Check sheet for the modelled part. Datum: model origin and axes. Units: mm. Round coordinates to 2 decimals unless told otherwise and drop trailing zeros. Write each loop counter-clockwise with the first axis right and the second up, starting at its lowest first coordinate (ties: lowest second). Pieces come first, ordered by that corner, then holes. Notation, with made-up numbers: (56.25, -26) -> (67.25, -26) arc R29 cw to (67.25, 3) -> close; hole circle Ø5 at (19.5, -17). An arc over 180 degrees is marked (long way). One line per item, written item: value.
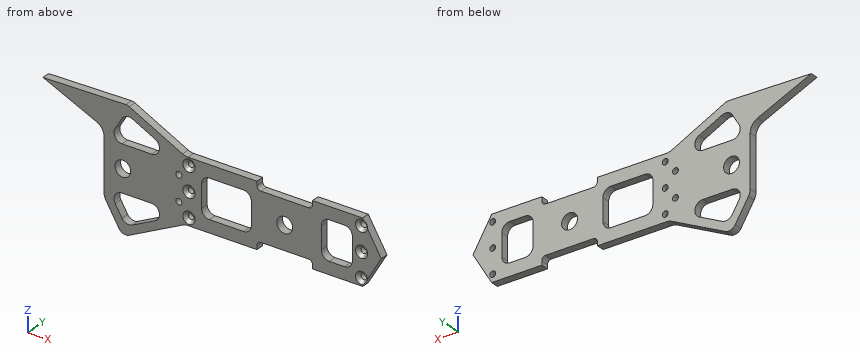
from build123d import *

# Parameters (mm, degrees)
CROQUIS1_R              = 6.35
SALIENTE_EXTRUIR1_DEPTH = 6.35
REDONDEO1_R             = 10
CORTAR_EXTRUIR2_DEPTH   = 225.405229946
CORTAR_EXTRUIR3_DEPTH   = 225.405229946
CROQUIS7_R              = 2.38125
CORTAR_EXTRUIR4_DEPTH   = 225.405229946
CROQUIS8_R              = 2.38125
CORTAR_EXTRUIR5_DEPTH   = 225.405229946
CHAFL_N1_SIZE           = 2.5


with BuildPart() as part:
    # Croquis1 → Saliente-Extruir1 (new body)
    with BuildSketch(Plane(origin=(0, 0, 0), x_dir=(1, 0, 0), z_dir=(0, 1, 0))):
        with BuildLine():
            Line((37.5, -25.4), (52.5, 0))
            Line((52.5, 0), (37.5, 25.4))
            Line((37.5, 25.4), (-105, 25.4))
            Line((-105, 25.4), (-149.746813481, 47.731727951))
            ThreePointArc((-149.746813481, 47.731727951), (-154.357530471, 48.146831931), (-158.024774803, 45.321528145))
            Line((-158.024774803, 45.321528145), (-170, 25.4))
            Line((-170, 25.4), (-170, -25.4))
            Line((-170, -25.4), (-219.03156103, -47.147007635))
            Line((-219.03156103, -47.147007635), (-152.702210171, -48.398869348))
            ThreePointArc((-152.702210171, -48.398869348), (-151.184140049, -48.244143221), (-149.746813481, -47.731727951))
            Line((-149.746813481, -47.731727951), (-105, -25.4))
            Line((-105, -25.4), (37.5, -25.4))
        make_face()
        with Locations(Location((-155, 0, 0), (0, 0, 270))):
            Circle(CROQUIS1_R, mode=Mode.SUBTRACT)
        with Locations(Location((-25, 0, 0), (0, 0, 270))):
            Circle(CROQUIS1_R, mode=Mode.SUBTRACT)
        with BuildLine():
            Line((-129.045100716, 30.303281185), (-147.329198773, 39.428299747))
            ThreePointArc((-147.329198773, 39.428299747), (-151.939915763, 39.843403727), (-155.607160095, 37.018099941))
            Line((-155.607160095, 37.018099941), (-161.092389512, 27.893081378))
            ThreePointArc((-161.092389512, 27.893081378), (-161.177056347, 21.495189828), (-155.65, 18.271553233))
            Line((-155.65, 18.271553233), (-131.880672526, 18.271553233))
            ThreePointArc((-131.880672526, 18.271553233), (-125.699998109, 23.164925706), (-129.045100716, 30.303281185))
        make_face(mode=Mode.SUBTRACT)
        with BuildLine():
            Line((-129.045100716, -30.303281185), (-147.329198773, -39.428299747))
            ThreePointArc((-147.329198773, -39.428299747), (-151.939915763, -39.843403727), (-155.607160095, -37.018099941))
            Line((-155.607160095, -37.018099941), (-161.092389512, -27.893081378))
            ThreePointArc((-161.092389512, -27.893081378), (-161.177056347, -21.495189828), (-155.65, -18.271553233))
            Line((-155.65, -18.271553233), (-131.880672526, -18.271553233))
            ThreePointArc((-131.880672526, -18.271553233), (-125.699998109, -23.164925706), (-129.045100716, -30.303281185))
        make_face(mode=Mode.SUBTRACT)
    extrude(amount=SALIENTE_EXTRUIR1_DEPTH)

    # Redondeo1
    redondeo1_edges = [part.edges().sort_by_distance(p)[0] for p in [
        (-105, 3.175, -25.4),
        (-170, 3.175, -25.4),
        (-170, 3.175, 25.4),
        (-105, 3.175, 25.4),
    ]]
    fillet(redondeo1_edges, radius=REDONDEO1_R)

    # Croquis5 → Cortar-Extruir2 (cut, through all)
    with BuildSketch(Plane.XZ):
        with BuildLine():
            Line((-5.875, 19.05), (-44.125, 19.05))
            ThreePointArc((-44.125, 19.05), (-46.37006403, 19.97993597), (-47.3, 22.225))
            Line((-47.3, 22.225), (-47.3, 25.4))
            Line((-47.3, 25.4), (-44.125, 25.4))
            Line((-44.125, 25.4), (-5.875, 25.4))
            Line((-5.875, 25.4), (-2.7, 25.4))
            Line((-2.7, 25.4), (-2.7, 22.225))
            ThreePointArc((-2.7, 22.225), (-3.62993597, 19.97993597), (-5.875, 19.05))
        make_face()
        with BuildLine():
            Line((-5.875, -19.05), (-44.125, -19.05))
            ThreePointArc((-44.125, -19.05), (-46.37006403, -19.97993597), (-47.3, -22.225))
            Line((-47.3, -22.225), (-47.3, -25.4))
            Line((-47.3, -25.4), (-44.125, -25.4))
            Line((-44.125, -25.4), (-5.875, -25.4))
            Line((-5.875, -25.4), (-2.7, -25.4))
            Line((-2.7, -25.4), (-2.7, -22.225))
            ThreePointArc((-2.7, -22.225), (-3.62993597, -19.97993597), (-5.875, -19.05))
        make_face()
    extrude(amount=-CORTAR_EXTRUIR2_DEPTH, mode=Mode.SUBTRACT)

    # Croquis6 → Cortar-Extruir3 (cut, through all)
    with BuildSketch(Plane.XZ):
        with BuildLine():
            Line((-85.475, 15.4), (-58.175, 15.4))
            ThreePointArc((-58.175, 15.4), (-53.684871939, 13.540128061), (-51.825, 9.05))
            Line((-51.825, 9.05), (-51.825, -9.05))
            ThreePointArc((-51.825, -9.05), (-53.684871939, -13.540128061), (-58.175, -15.4))
            Line((-58.175, -15.4), (-85.475, -15.4))
            ThreePointArc((-85.475, -15.4), (-89.965128061, -13.540128061), (-91.825, -9.05))
            Line((-91.825, -9.05), (-91.825, 9.05))
            ThreePointArc((-91.825, 9.05), (-89.965128061, 13.540128061), (-85.475, 15.4))
        make_face()
        with BuildLine():
            Line((10.675, 15.4), (22.975, 15.4))
            ThreePointArc((22.975, 15.4), (27.465128061, 13.540128061), (29.325, 9.05))
            Line((29.325, 9.05), (29.325, -9.05))
            ThreePointArc((29.325, -9.05), (27.465128061, -13.540128061), (22.975, -15.4))
            Line((22.975, -15.4), (10.675, -15.4))
            ThreePointArc((10.675, -15.4), (6.184871939, -13.540128061), (4.325, -9.05))
            Line((4.325, -9.05), (4.325, 9.05))
            ThreePointArc((4.325, 9.05), (6.184871939, 13.540128061), (10.675, 15.4))
        make_face()
    extrude(amount=-CORTAR_EXTRUIR3_DEPTH, mode=Mode.SUBTRACT)

    # Croquis7 → Cortar-Extruir4 (cut, through all)
    with BuildSketch(Plane.XZ):
        with Locations(Location((-101.825, 0, 0), (0, 0, 270))):
            Circle(CROQUIS7_R)
        with Locations(Location((-101.825, 19.4, 0), (0, 0, 270))):
            Circle(CROQUIS7_R)
        with Locations(Location((-101.825, -19.4, 0), (0, 0, 270))):
            Circle(CROQUIS7_R)
        with Locations(Location((36.675, -19.4, 0), (0, 0, 270))):
            Circle(CROQUIS7_R)
        with Locations(Location((36.675, 19.4, 0), (0, 0, 270))):
            Circle(CROQUIS7_R)
        with Locations(Location((36.675, 0, 0), (0, 0, 270))):
            Circle(CROQUIS7_R)
    extrude(amount=-CORTAR_EXTRUIR4_DEPTH, mode=Mode.SUBTRACT)

    # Croquis8 → Cortar-Extruir5 (cut, through all)
    with BuildSketch(Plane.XZ):
        with Locations(Location((-110, -10, 0), (0, 0, 270))):
            Circle(CROQUIS8_R)
        with Locations(Location((-110, 10, 0), (0, 0, 270))):
            Circle(CROQUIS8_R)
    extrude(amount=-CORTAR_EXTRUIR5_DEPTH, mode=Mode.SUBTRACT)

    # Chaflán1
    # the kernel refuses this chamfer: 2.5 mm, written as the material it takes off along each edge
    with BuildSketch(Plane(origin=(-101.825, 0, 19.4), x_dir=(0, 0, -1), z_dir=(-1, 0, 0))) as chafl_n1_piece_1:
        Polygon((2.38125 + CHAFL_N1_SIZE, 0), (2.38125, -CHAFL_N1_SIZE), (2.38125, 0), align=None)
    revolve(axis=Axis((-101.825, 0, 19.4), (0, -1, 0)), mode=Mode.SUBTRACT)
    with BuildSketch(Plane(origin=(36.675, 0, 19.4), x_dir=(0, 0, -1), z_dir=(-1, 0, 0))) as chafl_n1_piece_2:
        Polygon((2.38125 + CHAFL_N1_SIZE, 0), (2.38125, -CHAFL_N1_SIZE), (2.38125, 0), align=None)
    revolve(axis=Axis((36.675, 0, 19.4), (0, -1, 0)), mode=Mode.SUBTRACT)
    with BuildSketch(Plane(origin=(-101.825, 0, 0), x_dir=(0, 0, -1), z_dir=(-1, 0, 0))) as chafl_n1_piece_3:
        Polygon((2.38125 + CHAFL_N1_SIZE, 0), (2.38125, -CHAFL_N1_SIZE), (2.38125, 0), align=None)
    revolve(axis=Axis((-101.825, 0, 0), (0, -1, 0)), mode=Mode.SUBTRACT)
    with BuildSketch(Plane(origin=(-101.825, 0, -19.4), x_dir=(0, 0, -1), z_dir=(-1, 0, 0))) as chafl_n1_piece_4:
        Polygon((2.38125 + CHAFL_N1_SIZE, 0), (2.38125, -CHAFL_N1_SIZE), (2.38125, 0), align=None)
    revolve(axis=Axis((-101.825, 0, -19.4), (0, -1, 0)), mode=Mode.SUBTRACT)
    with BuildSketch(Plane(origin=(36.675, 0, 0), x_dir=(0, 0, -1), z_dir=(-1, 0, 0))) as chafl_n1_piece_5:
        Polygon((2.38125 + CHAFL_N1_SIZE, 0), (2.38125, -CHAFL_N1_SIZE), (2.38125, 0), align=None)
    revolve(axis=Axis((36.675, 0, 0), (0, -1, 0)), mode=Mode.SUBTRACT)
    with BuildSketch(Plane(origin=(36.675, 0, -19.4), x_dir=(0, 0, -1), z_dir=(-1, 0, 0))) as chafl_n1_piece_6:
        Polygon((2.38125 + CHAFL_N1_SIZE, 0), (2.38125, -CHAFL_N1_SIZE), (2.38125, 0), align=None)
    revolve(axis=Axis((36.675, 0, -19.4), (0, -1, 0)), mode=Mode.SUBTRACT)


solid = part.part
Item 1: Sectioned sample at C-C on y = 3.75. Count the separate pieces of the cut face and the enclosed holes in it, and give its area (3 significant figures).
Answer:
separate pieces: 1
enclosed holes: 14
area: 9,200 mm^2
Item 2: Sectioned sample at B-B on x = -110. Enter the section's corners in (y, z), and give its area (3 significant figures).
Answer:
outline: (0, -27.9) -> (6.35, -27.9) -> (6.35, -12.38) -> (0, -12.38) -> close; (0, -7.62) -> (6.35, -7.62) -> (6.35, 7.62) -> (0, 7.62) -> close; (0, 12.38) -> (6.35, 12.38) -> (6.35, 27.9) -> (0, 27.9) -> close
area: 294 mm^2
Item 3: Thickness scan on line 1 (X direction, y = 3.5, z = 3.5) (3 decimals); line 2 (X direction, y = 1.5, z = -20.5); line 3 (Z direction, x = -156.5, y = 3). Record the ranges inside material, lowest first.
Answer:
line 1: x = -170 to -160.298, -149.702 to -91.825, -51.825 to -30.298, -19.702 to 4.325, 29.325 to 50.433
line 2: x = -170 to -160.48, -127.05 to -105.02, -98.63 to -46.79, -3.21 to 33.48, 39.87 to 40.39
line 3: z = -47.05 to -35.53, -18.33 to -6.17, 6.17 to 18.33, 35.53 to 48.33
Item 4: Sectioned sample at A-A on x = -78.5. Enter the section's corners in (y, z), and give its area (3 significant figures).
Answer:
outline: (0, -25.4) -> (6.35, -25.4) -> (6.35, -15.4) -> (0, -15.4) -> close; (0, 15.4) -> (6.35, 15.4) -> (6.35, 25.4) -> (0, 25.4) -> close
area: 127 mm^2
Item 5: Depth check by flat-ended pin: P1, Ø3, axis at y = 1.5, z = 22, coming from the +X side; P2, Ø3, axis at y = 5, z = -7.5, coming from the +X side; P3, Ø4, axis at x = -14, z = -12, coming from the -Y side; P4, Ø2, axis at y = 3, z = -31, coming from the +X side. Enter the tip coordinate at first touch or a pass-through.
Answer:
P1: stops at x = 40.39
P2: stops at x = 48.96
P3: stops at y = 0
P4: stops at x = -114.22
